Input: part model. Units: mm. Frame: model coordinates. Face numbers are marked on the shaded views. A direction names the side the tool comes from. Coordinates: 2 decimals unless noted, no trailing zeros. Loops run counter-clockwise (first coordinate to the right, second up) from the corner with the lowest first, then second, coordinate; pieces in that order, holes last. Notation, with made-up numbers: (29.5, 25.5) -> (77.5, 25.5) arc R17 cw to (77.5, 36.5) -> close; hole circle Ø3 at (38.25, 22). An arc over 180 degrees is marked (long way). Answer as a JSON object with one key per item and string values.
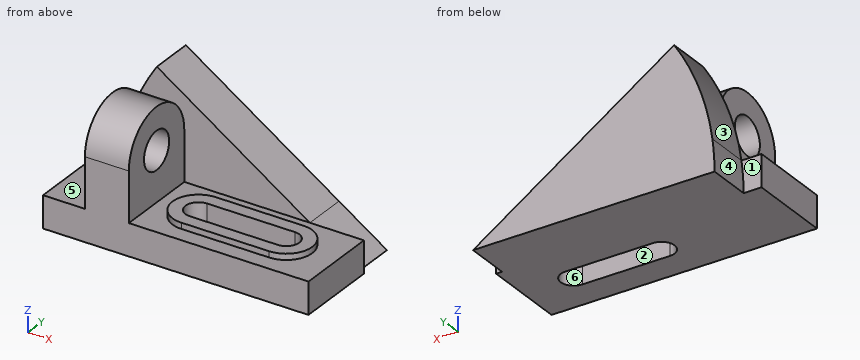
from build123d import *

# Parameters (mm, degrees)
F0_W      = 42
F0_H      = 16
F1_DEPTH  = 90
F3_DEPTH  = 22
F4_W      = 42
F4_H      = 16
F5_DEPTH  = 21
F7_DEPTH  = 3
F8_W      = 44
F8_H      = 13
F9_DEPTH  = 19
F11_DEPTH = 22


with BuildPart() as f1:
    # F0 (on Right) → F1 (new body)
    with BuildSketch(Plane.YZ):
        with Locations((24.0463, 16.209877)):
            Rectangle(F0_W, F0_H)
    extrude(amount=-F1_DEPTH)

    # F2 (on face) → F3 (join)
    with BuildSketch(Plane(origin=(-90, 0, 0), x_dir=(0, -1, 0), z_dir=(-1, 0, 0))):
        with BuildLine():
            Line((-45.0463, 49.209877), (-45.0463, 24.209877))
            Line((-45.0463, 24.209877), (-45.0463, 8.209877))
            Line((-45.0463, 8.209877), (-3.0463, 8.209877))
            Line((-3.0463, 8.209877), (-3.0463, 24.209877))
            Line((-3.0463, 24.209877), (-3.0463, 49.209877))
            Line((-3.0463, 49.209877), (-14.5463, 49.209877))
            ThreePointArc((-14.5463, 49.209877), (-24.0463, 39.709877), (-33.5463, 49.209877))
            Line((-33.5463, 49.209877), (-45.0463, 49.209877))
        make_face()
        with BuildLine():
            ThreePointArc((-3.0463, 49.209877), (-24.0463, 70.209877), (-45.0463, 49.209877))
            Line((-45.0463, 49.209877), (-33.5463, 49.209877))
            ThreePointArc((-33.5463, 49.209877), (-24.0463, 58.709877), (-14.5463, 49.209877))
            Line((-14.5463, 49.209877), (-3.0463, 49.209877))
        make_face()
    extrude(amount=F3_DEPTH)

    # F4 (on face) → F5 (join)
    with BuildSketch(Plane(origin=(-112, 0, 0), x_dir=(0, -1, 0), z_dir=(-1, 0, 0))):
        with Locations((-24.0463, 16.209877)):
            Rectangle(F4_W, F4_H)
    extrude(amount=F5_DEPTH)

    # F6 (on face) → F7 (join)
    with BuildSketch(Plane.XY.offset(24.209877)):
        with BuildLine():
            Line((-69, 11.0463), (-25, 11.0463))
            ThreePointArc((-25, 11.0463), (-12, 24.0463), (-25, 37.0463))
            Line((-25, 37.0463), (-69, 37.0463))
            ThreePointArc((-69, 37.0463), (-82, 24.0463), (-69, 11.0463))
        make_face()
    extrude(amount=F7_DEPTH)

    # F8 (on face) → F9 (cut)
    with BuildSketch(Plane.XY.offset(27.209877)):
        with Locations((-47, 24.0463)):
            Rectangle(F8_W, F8_H)
        with BuildLine():
            Line((-69, 17.5463), (-69, 30.5463))
            ThreePointArc((-69, 30.5463), (-75.5, 24.0463), (-69, 17.5463))
        make_face()
        with BuildLine():
            ThreePointArc((-25, 17.5463), (-18.5, 24.0463), (-25, 30.5463))
            Line((-25, 30.5463), (-25, 17.5463))
        make_face()
    extrude(amount=-F9_DEPTH, mode=Mode.SUBTRACT)

    # F10 (on face) → F11 (join)
    with BuildSketch(Plane(origin=(0, 45.0463, 0), x_dir=(-1, 0, 0), z_dir=(0, 1, 0))):
        with BuildLine():
            ThreePointArc((122.937484, 24.209877), (116.255949, 50.802013), (103.758959, 75.207132))
            Line((103.758959, 75.207132), (27.062827, 24.209877))
            Line((27.062827, 24.209877), (90, 24.209877))
            Line((90, 24.209877), (90, 49.209877))
            Line((90, 49.209877), (112, 49.209877))
            Line((112, 49.209877), (112, 24.209877))
            Line((112, 24.209877), (122.937484, 24.209877))
        make_face()
        with BuildLine():
            ThreePointArc((124, 8.209877), (123.734079, 16.227497), (122.937484, 24.209877))
            Line((122.937484, 24.209877), (112, 24.209877))
            Line((112, 24.209877), (112, 49.209877))
            Line((112, 49.209877), (90, 49.209877))
            Line((90, 49.209877), (90, 24.209877))
            Line((90, 24.209877), (27.062827, 24.209877))
            Line((27.062827, 24.209877), (3, 8.209877))
            Line((3, 8.209877), (124, 8.209877))
        make_face()
    extrude(amount=F11_DEPTH)


solid = f1.part
1. Section query D-D (z = 34.5). Return loops of the section in (x, y).
Reply:
{"outline": "(-121.11, 45.05) -> (-112, 45.05) -> (-112, 3.05) -> (-90, 3.05) -> (-90, 45.05) -> (-42.54, 45.05) -> (-42.54, 67.05) -> (-121.11, 67.05) -> close"}
2. Pin query (flat end, axial travel): P1, Ø24.5, axis at y = 24.05, z = 49.21, coming from the -X side; P2, Ø12.5, axis at x = -60.5, y = 18, coming from the +Z side; P3, Ø0.9, axis at x = -53, z = 26, coming from the -Y side. Return the tip coordinate at first contact, or that it passes through.
Reply:
{"P1": "stops at x = -112", "P2": "stops at z = 27.21", "P3": "stops at y = 11.05"}
3. Section query C-C (z = 52). Return loops of the section in (x, y), plus the area to 3 significant figures.
Reply:
{"outline": "(-115.8, 45.05) -> (-68.86, 45.05) -> (-68.86, 67.05) -> (-115.8, 67.05) -> close; (-112, 3.23) -> (-90, 3.23) -> (-90, 14.97) -> (-112, 14.97) -> close; (-112, 33.13) -> (-90, 33.13) -> (-90, 44.86) -> (-112, 44.86) -> close", "area": "1,550 mm2"}
4. Section query A-A (y = 26). Return loops of the section in (x, z), plus the area to 3 significant figures.
Reply:
{"outline": "(-133, 8.21) -> (-75.2, 8.21) -> (-75.2, 27.21) -> (-81.85, 27.21) -> (-81.85, 24.21) -> (-90, 24.21) -> (-90, 39.91) -> (-112, 39.91) -> (-112, 24.21) -> (-133, 24.21) -> close; (-112, 58.51) -> (-90, 58.51) -> (-90, 70.12) -> (-112, 70.12) -> close; (-18.8, 8.21) -> (0, 8.21) -> (0, 24.21) -> (-12.15, 24.21) -> (-12.15, 27.21) -> (-18.8, 27.21) -> close", "area": "1,870 mm2"}
5. Access query for the marked faces 4, 5 and 6. Directions: +Z, -Z, +X, -X, +Y, -Y. A direction counts if a zero-diameter tool reaches every point of the face in a straight line with its end or side. Return the directions, or none.
Reply:
{"face 4": "+Z, -X, +Y", "face 5": "+Z, -X, -Y", "face 6": "+Z, -Z"}
6. Section query B-B (x = -99). Return loops of the section in (y, z), plus the area to 3 significant figures.
Reply:
{"outline": "(3.05, 8.21) -> (67.05, 8.21) -> (67.05, 72.04) -> (45.05, 72.04) -> (45.05, 49.21) arc R21 ccw to (3.05, 49.21) -> close; hole circle Ø19 at (24.05, 49.21)", "area": "3,540 mm2"}
7. Mould query, pull axis X, two halves, no side actions, for the marked faces 1, 2 and 3. Classes: pulls with the +X half, pulls with the -X half, needs draft (parallel to the pull), parting line crosses it, or undercut.
Reply:
{"face 1": "needs draft", "face 2": "undercut", "face 3": "pulls with the -X half"}
8. Line query: line 1 along Y through (x, z) = (-28, 16.5); line 2 along Y through (x, z) = (-74, 45); line 3 along Z through (x, y) = (-82, 22). Output: solid intervals per line, ascending.
Reply:
{"line 1": "y = 3.05 to 17.55, 30.55 to 67.05", "line 2": "y = 45.05 to 67.05", "line 3": "z = 8.21 to 24.21"}
